```python
from build123d import *

# Parameters (mm, degrees)
SKETCH_1_R          = 15
EXTRUDE_1_DEPTH     = 20
CUT_EXTRUDE_1_DEPTH = 16.5
SKETCH_10_R         = 9
CUT_EXTRUDE_2_DEPTH = 24.5


with BuildPart() as part:
    # 草图1 → 凸台-拉伸1 (new body)
    with BuildSketch(Plane(origin=(0, 0, 0), x_dir=(1, 0, 0), z_dir=(0, 1, 0))):
        Circle(SKETCH_1_R)
    extrude(amount=EXTRUDE_1_DEPTH)

    # 草图2 → 切除-拉伸1 (cut, symmetric)
    with BuildSketch(Plane.XY):
        Polygon((-15, 5.786796564), (15, 18.213203436), (15, -10.377528432), (-15, -10.377528432), align=None)
    extrude(amount=CUT_EXTRUDE_1_DEPTH, both=True, mode=Mode.SUBTRACT)

    # 草图10 → 切除-拉伸2 (cut)
    with BuildSketch(Plane(origin=(0, 20, 0), x_dir=(1, 0, 0), z_dir=(0, 1, 0))):
        Circle(SKETCH_10_R)
    extrude(amount=-CUT_EXTRUDE_2_DEPTH, mode=Mode.SUBTRACT)


solid = part.part
```
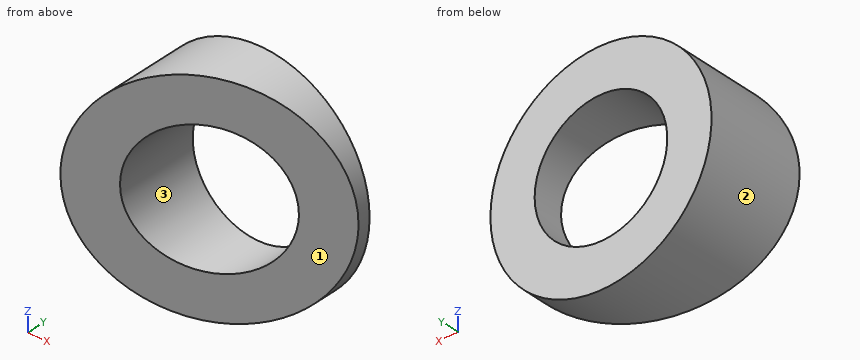
For this review, take the finished solid that the model builds, in its own axes (mm). Face numbers are marked on the shaded views. Give positions to 0.01 mm unless a question says otherwise; leave off trailing zeros. Order: outer loops, then holes, each group sorted by start corner. A loop starts at its lowest first (then second) coordinate and runs counter-clockwise, first axis right, second up.
1) The part is to be moulded in two halves that separate along X. For the marked faces 1, 2 and 3, say which applies: released by +X, released by -X, zero draft, split by the parting line, or undercut.
2) Take a section at B-B (z = 0). Give the boundary of the cut face in (x, y), then the cut area to 3 significant figures.
3) Take a section at A-A (x = 0). Give the boundary of the cut face in (y, z).
4) Take a section at D-D (x = 13). Give the boundary of the cut face in (y, z).
5) Wall thickness on line 1 (Z direction, x = 0, y = 15); line 2 (Z direction, x = -12, y = 14); line 3 (X direction, y = 16.25, z = 0): over which ranges is each line inside the solid? List them lowest first.
6) Insertion check: pin 1 (4 mm diameter, centred on x = -4.5, z = -5, fed in from +Y); pin 2 (4 mm diameter, centred on x = 11.5, z = -6, fed in from -Y) (3 decimals); pin 3 (8 mm diameter, centred on x = -8, y = 18.5, fed in from -Z); pin 4 (8 mm diameter, centred on y = 12.5, z = 9, fed in from -X). Each pin has a flat end and moves straight along its axis. Give the tip position at first contact, or say it passes through.
7) Take a section at C-C (y = 13.25). Give the boundary of the cut face in (x, z).
Derived:
1. face 1: released by +X
1. face 2: split by the parting line
1. face 3: undercut
2. outline: (-15, 5.79) - (-9, 8.27) - (-9, 20) - (-15, 20) - close; (9, 15.73) - (15, 18.21) - (15, 20) - (9, 20) - close
2. area: 96.0 mm2
3. outline: (12, -15) - (20, -15) - (20, -9) - (12, -9) - close; (12, 9) - (20, 9) - (20, 15) - (12, 15) - close
4. outline: (17.38, -7.48) - (20, -7.48) - (20, 7.48) - (17.38, 7.48) - close
5. line 1: z = -15 to -9, 9 to 15
5. line 2: z = -9 to 9
5. line 3: x = -15 to -9, 9 to 10.26
6. pin 1: passes through
6. pin 2: stops at y = 15.935
6. pin 3: stops at z = -14.46
6. pin 4: stops at x = -14.14
7. outline: (3.02, -14.69) - (3.02, -8.48) arc R9 cw (long way) to (3.02, 8.48) - (3.02, 14.69) arc R15 ccw (long way) to start
